Input: part model. Units: mm. Frame: model coordinates. A direction names the side the tool comes from. Round coordinates to 2 decimals unless told otherwise and drop trailing zeros. Loops run counter-clockwise (first coordinate to the right, second up) from the corner with the lowest first, then second, coordinate; pieces in that order, holes last.
(1) Cut plane C-C, the plane y = 30. Output: boundary loops of the cut face in (x, z), and give its area (3 significant figures).
(2) First-contact query: pin 1 Ø1.5 at (y, z) = (-5, -0.5) entering from +X; pin 2 Ø8 at (y, z) = (31.5, -5.5) entering from -X; pin 3 Ø6 at (x, y) = (-7, 2) entering from -Z; pin 4 Ø1 at (x, z) = (-4.5, 0) entering from +Y. Flat tips, straight axial feed; report the tip coordinate or a pass-through.
(3) Draft query along X for faces 4 (the face through (0.875, 38, 0)), 5 (the face through (-2.17, 0.27, 9.76)), 6 (the face through (-1.3, 39, 0)), 7 (the face through (-0.875, 38, 0)). Return one class per face: released by +X, released by -X, zero draft, split by the parting line, or undercut.
(4) Access query for faces 1 (the face through (1.3, 39, 0)), 2 (the face through (2, 27, 1)), 3 (the face through (0, 36.918, 0)). Directions: +Z, -Z, +X, -X, +Y, -Y. A direction counts if a zero-diameter tool reaches every point of the face in a straight line with its end or side. Return the directions, or none.
(5) Cut plane B-B, the plane z = 0. Output: boundary loops of the cut face in (x, y), and give its area (3 significant figures).
(6) Cut plane D-D, the plane z = 2.75. Output: boundary loops of the cut face in (x, y).
(7) Line query: line 1 (Y direction, x = -6.5, z = -3.75); line 2 (X direction, y = 19.5, z = 3.75); line 3 (Z direction, x = -8.75, y = -14). Output: solid intervals per line, ascending.
(8) Cut plane A-A, the plane x = 0. Output: boundary loops of the cut face in (y, z), and give its area (3 significant figures).
from build123d import *

# Parameters (mm, degrees)
SKETCH1_R               = 10
BOSS_EXTRUDE1_DEPTH     = 19
SKETCH2_R               = 4.25
BOSS_EXTRUDE2_DEPTH     = 8
SKETCH3_R               = 2
BOSS_EXTRUDE3_DEPTH     = 12
SKETCH4_W               = 1.75006174
SKETCH4_H               = 4.164275762
CUT_EXTRUDE1_DEPTH      = 11
CUT_EXTRUDE1_DEPTH_BACK = 11


with BuildPart() as part:
    # Sketch1 → Boss-Extrude1 (new body, symmetric)
    with BuildSketch(Plane(origin=(0, 0, 0), x_dir=(1, 0, 0), z_dir=(0, 1, 0))):
        Circle(SKETCH1_R)
    extrude(amount=BOSS_EXTRUDE1_DEPTH, both=True)

    # Sketch2 → Boss-Extrude2 (add)
    with BuildSketch(Plane(origin=(0, 19, 0), x_dir=(1, 0, 0), z_dir=(0, 1, 0))):
        Circle(SKETCH2_R)
    extrude(amount=BOSS_EXTRUDE2_DEPTH)

    # Sketch3 → Boss-Extrude3 (add)
    with BuildSketch(Plane(origin=(0, 27, 0), x_dir=(1, 0, 0), z_dir=(0, 1, 0))):
        Circle(SKETCH3_R)
    extrude(amount=BOSS_EXTRUDE3_DEPTH)

    # Sketch4 → Cut-Extrude1 (cut, two sides)
    with BuildSketch(Plane.XY) as cut_extrude1_sk:
        with Locations((0, 39)):
            Rectangle(SKETCH4_W, SKETCH4_H)
    extrude(amount=CUT_EXTRUDE1_DEPTH, mode=Mode.SUBTRACT)
    extrude(cut_extrude1_sk.sketch, amount=-CUT_EXTRUDE1_DEPTH_BACK, mode=Mode.SUBTRACT)


solid = part.part
Reported:
1. outline: circle Ø4 at (0, 0)
1. area: 12.6 mm2
2. pin 1: stops at x = 10
2. pin 2: stops at x = -1.32
2. pin 3: stops at z = -9.17
2. pin 4: stops at y = 27
3. face 4: undercut
3. face 5: split by the parting line
3. face 6: zero draft
3. face 7: undercut
4. face 1: +Z, -Z, +X, -X, +Y
4. face 2: +Y
4. face 3: +Z, -Z, +Y
5. outline: (-10, -19) - (10, -19) - (10, 19) - (4.25, 19) - (4.25, 27) - (2, 27) - (2, 39) - (0.88, 39) - (0.88, 36.92) - (-0.88, 36.92) - (-0.88, 39) - (-2, 39) - (-2, 27) - (-4.25, 27) - (-4.25, 19) - (-10, 19) - close
5. area: 872 mm2
6. outline: (-9.61, -19) - (9.61, -19) - (9.61, 19) - (3.24, 19) - (3.24, 27) - (-3.24, 27) - (-3.24, 19) - (-9.61, 19) - close
7. line 1: y = -19 to 19
7. line 2: x = -2 to 2
7. line 3: z = -4.84 to 4.84
8. outline: (-19, -10) - (19, -10) - (19, -4.25) - (27, -4.25) - (27, -2) - (36.92, -2) - (36.92, 2) - (27, 2) - (27, 4.25) - (19, 4.25) - (19, 10) - (-19, 10) - close
8. area: 868 mm2
